from build123d import *

# Parameters (mm, degrees)
F0_W     = 50
F0_H     = 50
F1_DEPTH = 50
F2_R     = 15
F3_DEPTH = 50
F4_DEPTH = 50


with BuildPart() as f1:
    # F0 (on Top) → F1 (new body)
    with BuildSketch(Plane.XY):
        Rectangle(F0_W, F0_H)
    extrude(amount=F1_DEPTH)

    # F2 (on face) → F3 (cut)
    with BuildSketch(Plane.XY.offset(50)):
        Circle(F2_R)
    extrude(amount=-F3_DEPTH, mode=Mode.SUBTRACT)

    # F4 (add): a face of the model
    f4_faces = [f1.faces().sort_by_distance(p)[0] for p in [
        (0, 24.2928932188, 50),
    ]]
    extrude(f4_faces, amount=F4_DEPTH)


solid = f1.part
Could you check a few things on this model? Use its own coordinates, in mm. Coordinates: 2 decimals unless noted, no trailing zeros. Order: outer loops, then holes, each group sorted by start corner. A loop starts at its lowest first (then second) coordinate and runs counter-clockwise, first axis right, second up.
Q1. Suppose I cut it at C-C on z = 47.5. Please give me the cut outline in (x, y).
Q2. Thinking about a two-plate mould opening in Y: for faces 1 (the flat face through (25, 0, 49)), 2 (the flat face through (0, -25, 49)), 3 (the cylindrical face through (-14.985, 0.66, 49.3)), which applies, released by +Y, released by -Y, zero draft, split by the parting line, or undercut?
Q3. Please list where these lines run through material, in increasing order: L1, parallel to Y at x = 0, z = 32; L2, parallel to Y at x = 4, z = 40.5; L3, parallel to X at y = -4.5, z = 32.
Q4. Suppose I cut it at A-A on y = 0. Please give me the cut outline in (x, z), and give its area (3 significant figures).
Answer:
1. outline: (-25, -25) - (25, -25) - (25, 25) - (-25, 25) - close; hole circle Ø30 at (0, 0)
2. face 1: zero draft
2. face 2: released by -Y
2. face 3: undercut
3. L1: y = -25 to -15, 15 to 25
3. L2: y = -25 to -14.46, 14.46 to 25
3. L3: x = -25 to -14.31, 14.31 to 25
4. outline: (-25, 0) - (-15, 0) - (-15, 100) - (-25, 100) - close; (15, 0) - (25, 0) - (25, 100) - (15, 100) - close
4. area: 2,000 mm2
